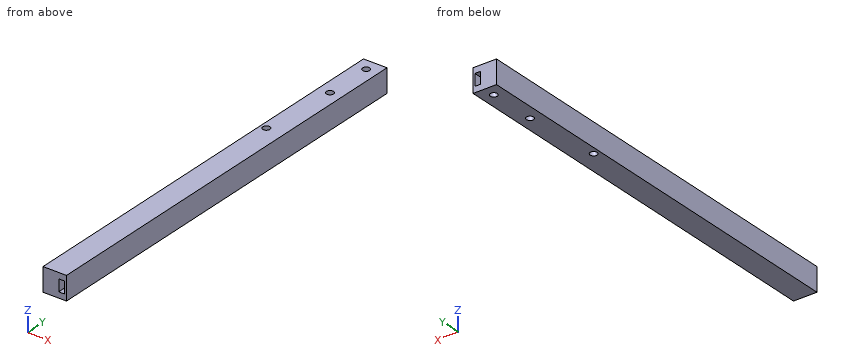
```python
from build123d import *

# Parameters (mm, degrees)
SKETCH_1_W         = 9.9
SKETCH_1_H         = 9.9
SKETCH_1_W_2       = 2.5
SKETCH_1_H_2       = 5
EXTRUDE_1_DEPTH    = 177
SKETCH2_R          = 1.5
CUT_EXTRUDE2_DEPTH = 10.9


with BuildPart() as part:
    # Эскиз1 → Бобышка-Вытянуть1 (new body)
    with BuildSketch(Plane(origin=(0, 0, 0), x_dir=(1, 0, 0), z_dir=(0, 1, 0))):
        with Locations((-0.744758221, -0.10825854)):
            Rectangle(SKETCH_1_W, SKETCH_1_H)
        with Locations((2.205241779, -0.10825854)):
            Rectangle(SKETCH_1_W_2, SKETCH_1_H_2, mode=Mode.SUBTRACT)
    extrude(amount=EXTRUDE_1_DEPTH)

    # Sketch2 → Cut-Extrude2 (cut, through all)
    with BuildSketch(Plane(origin=(0, 0, -4.84174146), x_dir=(-1, 0, 0), z_dir=(0, 0, -1))):
        with Locations((0.744758221, 172)):
            Circle(SKETCH2_R)
        with Locations((3.144758221, 120)):
            Circle(SKETCH2_R)
        with Locations((0.744758221, 152)):
            Circle(SKETCH2_R)
    extrude(amount=-CUT_EXTRUDE2_DEPTH, mode=Mode.SUBTRACT)


solid = part.part
```
Can you work these out from the model? Positions are in its coordinate system, mm. Give positions to 0.01 mm unless a question says otherwise; leave off trailing zeros. Order: outer loops, then holes, each group sorted by start corner. A loop starts at its lowest first (then second) coordinate and runs counter-clockwise, first axis right, second up. Notation, with made-up numbers: (40.25, -9.75) - (72.25, -9.75) arc R33 ccw to (72.25, 22.25) - close; hole circle Ø7 at (9.5, -22). An arc over 180 degrees is marked (long way). Use a Markdown table: item, result. Add a question column.
Q1. If we section it at A-A on y = 172: Write out the boundary of the cut face in (x, z), plus the area to 3 significant figures.
Q2. Please list where these lines run through material, in increasing order: line 1 along Y through (x, z) = (-0.5, -0.5); line 2 along X through (y, z) = (120, -0.75); line 3 along X through (y, z) = (172, 2.75).
Q3. If we section it at C-C on y = 56: Write out the boundary of the cut face in (x, z).
Q4. If we section it at B-B on z = 0.25: Write out the boundary of the cut face in (x, y), plus the area to 3 significant figures.
Answers follow:
| question | item | result |
|---|---|---|
| 1 | outline | (-5.69, -4.84) - (-2.24, -4.84) - (-2.24, 5.06) - (-5.69, 5.06) - close; (0.76, -4.84) - (4.21, -4.84) - (4.21, 5.06) - (0.76, 5.06) - close; hole (0.96, -2.39) - (3.46, -2.39) - (3.46, 2.61) - (0.96, 2.61) - close |
| 1 | area | 55.8 mm^2 |
| 2 | line 1 | y = 0 to 150.52, 153.48 to 170.52, 173.48 to 177 |
| 2 | line 2 | x = -5.69 to -4.64, -1.64 to 0.96, 3.46 to 4.21 |
| 2 | line 3 | x = -5.69 to -2.24, 0.76 to 4.21 |
| 3 | outline | (-5.69, -4.84) - (4.21, -4.84) - (4.21, 5.06) - (-5.69, 5.06) - close; hole (0.96, -2.39) - (3.46, -2.39) - (3.46, 2.61) - (0.96, 2.61) - close |
| 4 | outline | (-5.69, 0) - (0.96, 0) - (0.96, 177) - (-5.69, 177) - close; (3.46, 0) - (4.21, 0) - (4.21, 177) - (3.46, 177) - close; hole circle Ø3 at (-3.14, 120); hole circle Ø3 at (-0.74, 152); hole circle Ø3 at (-0.74, 172) |
| 4 | area | 1,290 mm^2 |
